from build123d import *

# Parameters (mm, degrees)
SKETCH1_R           = 2.55
SKETCH1_R_2         = 3.6
BOSS_EXTRUDE1_DEPTH = 3


with BuildPart() as part:
    # Sketch1 → Boss-Extrude1 (new body)
    with BuildSketch(Plane(origin=(0, 0, 0), x_dir=(1, 0, 0), z_dir=(0, 1, 0))):
        with BuildLine():
            Line((29.75, -32.75), (-29.75, -32.75))
            ThreePointArc((-29.75, -32.75), (-31.871320344, -31.871320344), (-32.75, -29.75))
            Line((-32.75, -29.75), (-32.75, 29.75))
            ThreePointArc((-32.75, 29.75), (-31.871320344, 31.871320344), (-29.75, 32.75))
            Line((-29.75, 32.75), (29.75, 32.75))
            ThreePointArc((29.75, 32.75), (31.871320344, 31.871320344), (32.75, 29.75))
            Line((32.75, 29.75), (32.75, -29.75))
            ThreePointArc((32.75, -29.75), (31.871320344, -31.871320344), (29.75, -32.75))
        make_face()
        with Locations((0, 10)):
            Circle(SKETCH1_R, mode=Mode.SUBTRACT)
        Circle(SKETCH1_R, mode=Mode.SUBTRACT)
        with Locations((10, 0)):
            Circle(SKETCH1_R, mode=Mode.SUBTRACT)
        with Locations((-10, 0)):
            Circle(SKETCH1_R, mode=Mode.SUBTRACT)
        with Locations((-19.85, 20)):
            Circle(SKETCH1_R_2, mode=Mode.SUBTRACT)
        with Locations((-19.85, 0)):
            Circle(SKETCH1_R_2, mode=Mode.SUBTRACT)
        with Locations((-19.85, -20)):
            Circle(SKETCH1_R_2, mode=Mode.SUBTRACT)
        with Locations((-19.85, 10)):
            Circle(SKETCH1_R, mode=Mode.SUBTRACT)
        with Locations((19.85, 20)):
            Circle(SKETCH1_R, mode=Mode.SUBTRACT)
        with Locations((19.85, 0)):
            Circle(SKETCH1_R, mode=Mode.SUBTRACT)
        with Locations((19.85, -20)):
            Circle(SKETCH1_R, mode=Mode.SUBTRACT)
        with Locations((0, -10)):
            Circle(SKETCH1_R, mode=Mode.SUBTRACT)
        with Locations((19.85, 10)):
            Circle(SKETCH1_R, mode=Mode.SUBTRACT)
        with Locations((19.85, -10)):
            Circle(SKETCH1_R, mode=Mode.SUBTRACT)
        with Locations((-19.85, -10)):
            Circle(SKETCH1_R, mode=Mode.SUBTRACT)
        with BuildLine():
            Line((10.32, 17.5), (-10.32, 17.5))
            ThreePointArc((-10.32, 17.5), (-12.82, 20), (-10.32, 22.5))
            Line((-10.32, 22.5), (10.32, 22.5))
            ThreePointArc((10.32, 22.5), (12.82, 20), (10.32, 17.5))
        make_face(mode=Mode.SUBTRACT)
        with BuildLine():
            Line((3.25, 26.2), (-3.25, 26.2))
            ThreePointArc((-3.25, 26.2), (-4.75, 27.7), (-3.25, 29.2))
            Line((-3.25, 29.2), (3.25, 29.2))
            ThreePointArc((3.25, 29.2), (4.75, 27.7), (3.25, 26.2))
        make_face(mode=Mode.SUBTRACT)
        with BuildLine():
            Line((-16.9, 26.2), (-23.4, 26.2))
            ThreePointArc((-23.4, 26.2), (-24.9, 27.7), (-23.4, 29.2))
            Line((-23.4, 29.2), (-16.9, 29.2))
            ThreePointArc((-16.9, 29.2), (-15.4, 27.7), (-16.9, 26.2))
        make_face(mode=Mode.SUBTRACT)
        with BuildLine():
            Line((16.9, 26.2), (23.4, 26.2))
            ThreePointArc((23.4, 26.2), (24.9, 27.7), (23.4, 29.2))
            Line((23.4, 29.2), (16.9, 29.2))
            ThreePointArc((16.9, 29.2), (15.4, 27.7), (16.9, 26.2))
        make_face(mode=Mode.SUBTRACT)
        with BuildLine():
            Line((10.32, -17.5), (-10.32, -17.5))
            ThreePointArc((-10.32, -17.5), (-12.82, -20), (-10.32, -22.5))
            Line((-10.32, -22.5), (10.32, -22.5))
            ThreePointArc((10.32, -22.5), (12.82, -20), (10.32, -17.5))
        make_face(mode=Mode.SUBTRACT)
        with BuildLine():
            Line((-16.9, -26.2), (-23.4, -26.2))
            ThreePointArc((-23.4, -26.2), (-24.9, -27.7), (-23.4, -29.2))
            Line((-23.4, -29.2), (-16.9, -29.2))
            ThreePointArc((-16.9, -29.2), (-15.4, -27.7), (-16.9, -26.2))
        make_face(mode=Mode.SUBTRACT)
        with BuildLine():
            Line((3.25, -26.2), (-3.25, -26.2))
            ThreePointArc((-3.25, -26.2), (-4.75, -27.7), (-3.25, -29.2))
            Line((-3.25, -29.2), (3.25, -29.2))
            ThreePointArc((3.25, -29.2), (4.75, -27.7), (3.25, -26.2))
        make_face(mode=Mode.SUBTRACT)
        with BuildLine():
            Line((16.9, -26.2), (23.4, -26.2))
            ThreePointArc((23.4, -26.2), (24.9, -27.7), (23.4, -29.2))
            Line((23.4, -29.2), (16.9, -29.2))
            ThreePointArc((16.9, -29.2), (15.4, -27.7), (16.9, -26.2))
        make_face(mode=Mode.SUBTRACT)
    extrude(amount=BOSS_EXTRUDE1_DEPTH)


solid = part.part
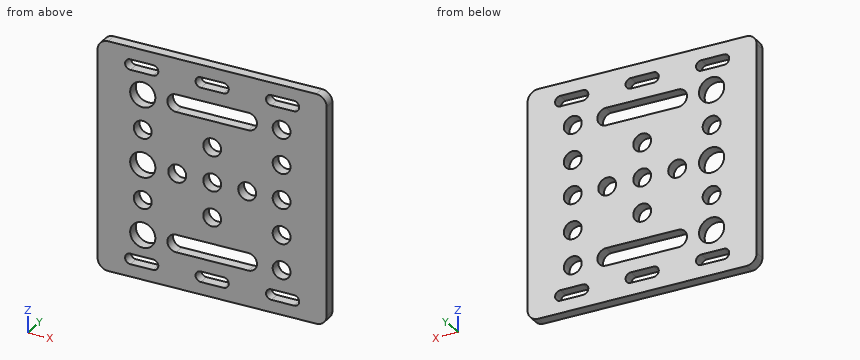
Source: CAD feature listing. Evaluate the final solid. Frame: model axes, mm. Coordinates: 2 decimals unless noted, no trailing zeros. Loops run counter-clockwise (first coordinate to the right, second up) from the corner with the lowest first, then second, coordinate; pieces in that order, holes last. Notation, with made-up numbers: M 36,58 L 90,58 A24 ccw 90,92 Z; hole C 37.5,56.5 d6. An arc over 180 degrees is marked long. Answer in a Markdown table with one row per item.
Q1. Section A-A on z = -20. Return the cut outline in (x, y).
Answers below:
| item | result |
|---|---|
| outline | M -32.75,0 L -23.45,0 L -23.45,3 L -32.75,3 Z; M -16.25,0 L -12.82,0 L -12.82,3 L -16.25,3 Z; M 12.82,0 L 17.3,0 L 17.3,3 L 12.82,3 Z; M 22.4,0 L 32.75,0 L 32.75,3 L 22.4,3 Z |
Q2. Section B-B on x = 19.85. State how many separate pieces and enclosed holes the cut face has, plus the area to 3 significant figures.
Answers below:
| item | result |
|---|---|
| separate pieces | 8 |
| enclosed holes | 0 |
| area | 102 mm^2 |
Q3. First-contact query: pin 1 (3 mm diameter, centred on x = 19.85, z = 0, fed in from +Y). Flat tip, straight axial feed; report the tip coordinate or a pass-through.
Answers below:
| item | result |
|---|---|
| pin 1 | passes through |
Q4. Ray query, probe 1 along X at (y, z) = (2.05, 0); probe 2 along Z at (x, y) = (-10, 2.4); probe 3 along Z at (x, y) = (23.5, 2.3). Return the intervals inside material, ascending. Write a range as from..to.
Answers below:
| item | result |
|---|---|
| probe 1 | x = -32.75..-23.45, -16.25..-12.55, -7.45..-2.55, 2.55..7.45, 12.55..17.3, 22.4..32.75 |
| probe 2 | z = -32.75..-22.5, -17.5..-2.55, 2.55..17.5, 22.5..32.75 |
| probe 3 | z = -32.75..-29.2, -26.2..26.2, 29.2..32.75 |
Q5. Section C-C on z = 27.7. Return the cut outline in (x, y).
Answers below:
| item | result |
|---|---|
| outline | M -32.75,0 L -24.9,0 L -24.9,3 L -32.75,3 Z; M -15.4,0 L -4.75,0 L -4.75,3 L -15.4,3 Z; M 4.75,0 L 15.4,0 L 15.4,3 L 4.75,3 Z; M 24.9,0 L 32.75,0 L 32.75,3 L 24.9,3 Z |
